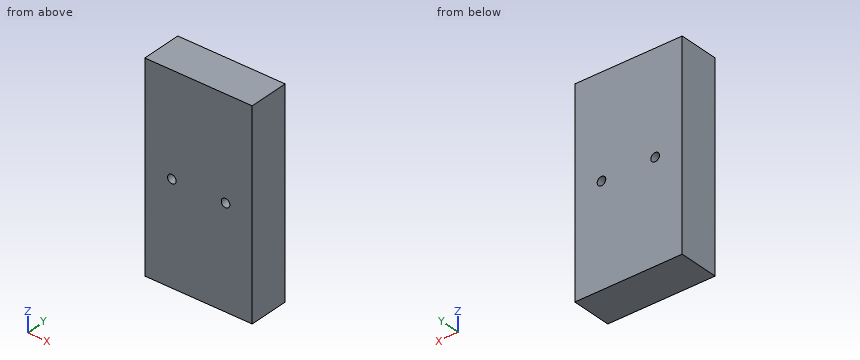
Autodesk Inventor part; units mm, degrees
ref_plane "YZ Plane" through (0, 0, 0) normal (1, 0, 0) x (0, 1, 0)
ref_plane "XZ Plane" through (0, 0, 0) normal (0, 1, 0) x (-1, 0, 0)
ref_plane "XY Plane" through (0, 0, 0) normal (0, 0, 1) x (1, 0, 0)
sketch "Эскиз1" plane through (0, 0, 0) normal (0, 1, 0) x (-1, 0, 0)
  line L0 (-20, 37.5) -> (20, 37.5)
  line L1 (20, 37.5) -> (20, -37.5)
  line L2 (20, -37.5) -> (-20, -37.5)
  line L3 (-20, -37.5) -> (-20, 37.5)
  line L4 (-20, 37.5) -> (20, -37.5) construction
  line L5 (20, 37.5) -> (-20, -37.5) construction
  point P0 (0, 0)
  dimension "d0" = 75
  dimension "d1" = 40
extrude "Выдавливание1" add sketch "Эскиз1" along normal blind 15
sketch "Эскиз2" plane through (0, 15, 0) normal (0, 1, 0) x (1, 0, 0)
  circle A0 centre (10.0691, 0) radius 1.6
  circle A1 centre (-9.9309, 0) radius 1.6
  line L0 (-9.9309, 0) -> (10.0691, 0)
  line L1 (20, 37.5) -> (-20, 37.5)
  line L2 (0, 37.5) -> (0, -37.5)
  line L3 (-20, -37.5) -> (20, -37.5)
  line L4 (-20, 37.5) -> (-20, -37.5)
  line L5 (-20, 0) -> (20.2069, 0)
  point P0 (0, 0)
  point P1 (0.0691, 0)
  dimension "d4" = 3.2
  dimension "d5" = 3.2
  dimension "d6" = 20
extrude "Выдавливание2" cut sketch "Эскиз2" against normal blind 15 contours L5 L0 A0 | A0 L0 L5 | L0 L5 A1 | A1 L5 L0
properties part number "холдер"
The listing builds one solid part. Answer for the finished solid, in the listing's coordinates (mm). Round coordinates to 2 decimals unless told otherwise and drop trailing zeros. Order: outer loops, then holes, each group sorted by start corner. A loop starts at its lowest first (then second) coordinate and runs counter-clockwise, first axis right, second up. Notation, with made-up numbers: (-8.75, 19) - (48.25, 19) arc R18 ccw to (48.25, 43) - close; hole circle Ø7 at (-22, 65). An arc over 180 degrees is marked (long way). Write item = value, one per line. Start each with the question number.
1) Straight lines are drawn through the part: L1, parallel to X at y = 10.75, z = 0; L2, parallel to Z at x = -9, y = 13.75; L3, parallel to Z at x = -8.5, y = 12. For each, find the intervals that lie inside material, in ascending order.
2) Given pin 1 (3.5 mm diameter, centred on x = 10.07, z = 0, fed in from +Y); pin 2 (1.9 mm diameter, centred on x = -9.93, z = 0, fed in from +Y), each flat-ended and moving along its own axis, determine where each tip first touches the part or whether it passes through.
3) Section A-A, the plane z = 0 is taken. Write down the section's boundary in (x, y), plus the area to 3 significant figures.
Results list:
q1.L1 = -20 to -11.53, -8.33 to 8.47, 11.67 to 20
q1.L2 = -37.5 to -1.3, 1.3 to 37.5
q1.L3 = -37.5 to -0.72, 0.72 to 37.5
q2.pin_1 = 15
q2.pin_2 = through
q3.outline = (-20, 0) - (-11.53, 0) - (-11.53, 15) - (-20, 15) - close; (-8.33, 0) - (8.47, 0) - (8.47, 15) - (-8.33, 15) - close; (11.67, 0) - (20, 0) - (20, 15) - (11.67, 15) - close
q3.area = 504 mm^2
